Autodesk Inventor part; units mm, degrees
ref_plane "YZ Plane" through (0, 0, 0) normal (1, 0, 0) x (0, 1, 0)
ref_plane "XZ Plane" through (0, 0, 0) normal (0, 1, 0) x (-1, 0, 0)
ref_plane "XY Plane" through (0, 0, 0) normal (0, 0, 1) x (1, 0, 0)
sketch "Sketch1" plane through (0, 0, 0) normal (0, 0, 1) x (1, 0, 0)
  line L0 (-34.925, -12.7) -> (34.925, -12.7)
  line L1 (34.925, -12.7) -> (34.925, 12.7)
  line L2 (34.925, 12.7) -> (-34.925, 12.7)
  line L3 (-34.925, 12.7) -> (-34.925, -12.7)
  line L4 (-34.925, -12.7) -> (34.925, 12.7) construction
  line L5 (34.925, -12.7) -> (-34.925, 12.7) construction
  point P0 (0, 0)
  dimension "d0" = 25.4
  dimension "d1" = 69.85
extrude "Extrusion1" add sketch "Sketch1" along normal blind 5.08
sketch "Sketch2" plane through (0, 0, 5.08) normal (0, 0, 1) x (1, 0, 0)
  line L0 (-34.925, 12.7) -> (-34.925, -12.7)
  line L1 (34.925, -12.7) -> (34.925, 12.7)
  line L2 (34.925, 12.7) -> (-34.925, 12.7)
  point P0 (0, 0)
  point P1 (3.175, 2.54)
  point P2 (22.225, 2.54)
  dimension "d5" = 12.7
  dimension "d6" = 10.16
  dimension "d7" = 10.16
  dimension "d18" = 19.05
hole "Hole1" at (3.175, 2.54, 5.08) at (22.225, 2.54, 5.08) direction (0, 0, -1) diameter 6.35 end through all
sketch "Sketch5" plane through (0, 0, 5.08) normal (0, 0, 1) x (1, 0, 0)
  line L0 (34.925, 12.7) -> (-34.925, 12.7)
  line L1 (-34.925, 12.7) -> (-14.2875, 12.7)
  line L2 (-14.2875, 12.7) -> (-14.2875, 3.81)
  line L3 (-14.2875, 3.81) -> (-34.925, 3.81)
  line L4 (-34.925, 3.81) -> (-34.925, 12.7)
  line L5 (-34.925, 12.7) -> (-34.925, -12.7)
  line L6 (-34.925, -12.7) -> (-14.2875, -12.7)
  line L7 (-14.2875, -12.7) -> (-14.2875, -3.81)
  line L8 (-14.2875, -3.81) -> (-34.925, -3.81)
  line L9 (-34.925, -3.81) -> (-34.925, -12.7)
  point P0 (0, 0)
  dimension "d19" = 7.62
extrude "Extrusion2" add sketch "Sketch5" along normal blind 10.16
sketch "Sketch7" plane through (0, 0, 5.08) normal (0, 0, 1) x (1, 0, 0)
  line L0 (-29.845, 3.81) -> (-34.925, 3.81)
  line L1 (-19.3675, -3.81) -> (-14.2875, -3.81)
  line L2 (-34.925, 3.81) -> (-14.2875, 3.81)
  line L3 (-14.2875, 3.81) -> (-14.2875, -3.81)
  line L4 (-14.2875, -3.81) -> (-34.925, -3.81)
  line L5 (-34.925, -3.81) -> (-34.925, 3.81)
  point P0 (0, 0)
extrude "Extrusion4" cut sketch "Sketch7" against normal blind 12.7
fillet "Fillet2" radius 5.08 2 edges at (-34.925, 8.255, 0) (-34.925, -8.255, 0)
sketch "Sketch8" plane through (34.925, -12.7, 0) normal (0, -1, 0) x (1, 0, 0)
  line L0 (-69.85, 5.08) -> (-69.85, 15.24)
  line L1 (-64.77, 0) -> (0, 0)
  point P0 (-34.925, 0)
  point P1 (-62.23, 7.62)
  point P2 (-69.85, 10.16)
  dimension "d28" = 7.62
  dimension "d29" = 7.62
hole "Hole2" at (-27.305, -12.7, 7.62) direction (0, 1, 0) diameter 5.08 end through all
sketch "Sketch9" plane through (34.925, 12.7, 5.08) normal (0, 1, 0) x (1, 0, 0)
  line L0 (-49.2125, -10.16) -> (-69.85, -10.16)
  line L1 (-69.85, -10.16) -> (-38.1, 0)
  line L2 (-49.2125, 0) -> (0, 0)
  line L3 (-38.1, -10.16) -> (-38.1, 0)
  line L4 (-38.1, -10.16) -> (-69.85, -10.16)
  line L5 (-38.1, 0) -> (-58.7375, 0)
  line L6 (-58.7375, 0) -> (-58.7375, -6.604)
  point P0 (-34.925, 5.08)
extrude "Extrusion5" cut sketch "Sketch9" against normal through all contours L0 L1 L3 L4
extrude "Extrusion6" add sketch "Sketch9" against normal up to surface (8.89 mm away) contours L6 L5 L2 L1
fillet "Fillet3" radius 5.08 1 edges at (-34.925, 8.255, 15.24)
fillet "Fillet4" radius 5.08 1 edges at (-34.925, -8.255, 15.24)
extrude "Extrusion7" add sketch "Sketch9" along normal up to surface (8.89 mm away) from surface at -25.4 contours L6 L5 L2 L1
fillet "Fillet5" radius 5.08 1 edges at (34.925, 0, 5.08)
fillet "Fillet6" radius 5.08 1 edges at (-14.2875, 0, 5.08)
properties part number "Upper_Spring_Hanger2"
Design review of the part built by this model. Coordinates are the model's own, in mm. Give positions to 0.01 mm unless a question says otherwise; leave off trailing zeros. Loops run counter-clockwise (first coordinate to the right, second up) from the corner with the lowest first, then second, coordinate; pieces in that order, holes last. Notation, with made-up numbers: M -27.75,42 L -13.75,42 A22 cw -13.75,76 Z; hole C 15,61.25 d2. An arc over 180 degrees is marked long. Return JSON: item names as keys, results as strings. Group by question number.
Item 1: We need section B-B (x = -22.5). Give the boundary of the cut face in (y, z).
Item 2: Mouldability with a two-part tool opening along Y and no side actions: class faces 1 (the cylindrical face through (-12.76, -0.05, 3.63)), 2 (the flat face through (-15.912, -8.193, 9.156)), 3 (the flat face through (-7, 12.7, 4)) as released by +Y, released by -Y, zero draft, split by the parting line, or undercut.
Item 3: For probe 1 along Y at (x, z) = (-17, 3.25); probe 2 along X at (y, z) = (2.54, 2); probe 3 along Z at (x, y) = (23, -3.75), list the stretches that pass through material, from the lowest coordinate up.
Item 4: We need section D-D (z = 3.25). Give the boundary of the cut face in (x, y) (3 decimals).
Item 5: Insertion check: pin 1 Ø4 at (x, y) = (23, 3.5) entering from +Z; pin 2 Ø4 at (x, z) = (-27.305, 7.62) entering from +Y; pin 3 Ø2 at (y, z) = (-9, 9.5) entering from -X; pin 4 Ø10 at (x, y) = (3.175, 2.54) entering from -Z. Each pin has a flat end and moves straight along its axis. Give the tip position at first contact, or say it passes through.
Item 6: We need section A-A (y = 2.54). Give the number of separate pieces and of enclosed holes in the cut face, and give its area (3 significant figures).
Output:
{
 "1": {"outline": "M -12.7,0 L -3.81,0 L -3.81,11.26 L -12.7,11.26 Z; M 3.81,0 L 12.7,0 L 12.7,11.26 L 3.81,11.26 Z"},
 "2": {"face 1": "undercut", "face 2": "zero draft", "face 3": "released by +Y"},
 "3": {"probe 1": "y = -12.7 to -3.81, 3.81 to 12.7", "probe 2": "x = -13.88 to 0, 6.35 to 19.05, 25.4 to 34.51", "probe 3": "z = 0 to 5.08"},
 "4": {"outline": "M -34.584,-12.7 L 33.749,-12.7 L 33.749,12.7 L -34.584,12.7 L -34.584,3.81 L -13.112,3.81 L -13.112,-3.81 L -34.584,-3.81 Z; hole C 3.175,2.54 d6.35; hole C 22.225,2.54 d6.35"},
 "5": {"pin 1": "stops at z = 5.08", "pin 2": "passes through", "pin 3": "stops at x = -34.92", "pin 4": "stops at z = 0"},
 "6": {"separate pieces": "3", "enclosed holes": "0", "area": "174 mm^2"}
}
